Here's how the part is built. I have some questions about the finished solid (model axes, mm). A direction names the side the tool comes from. Round coordinates to 2 decimals unless told otherwise and drop trailing zeros. Order: outer loops, then holes, each group sorted by start corner. A loop starts at its lowest first (then second) coordinate and runs counter-clockwise, first axis right, second up. Notation, with made-up numbers: M 52.5,60.5 L 110.5,60.5 A16 cw 110.5,83.5 Z; hole C 52.5,70.5 d9. An arc over 180 degrees is marked long. Use one line per item in the form item = value. Start each with the question number.
```python
from build123d import *

# Parameters (mm, degrees)
BOSS_EXTRUDE1_DEPTH = 42
SKETCH2_R           = 2
CUT_EXTRUDE2_DEPTH  = 52.578217301
CUT_EXTRUDE3_DEPTH  = 4
SKETCH4_R           = 2
CUT_EXTRUDE4_DEPTH  = 52.578217301
SKETCH5_R           = 2
CUT_EXTRUDE5_DEPTH  = 65.722484597


with BuildPart() as part:
    # Sketch1 → Boss-Extrude1 (new body)
    with BuildSketch(Plane(origin=(0, 0, 0), x_dir=(0, 0, -1), z_dir=(1, 0, 0))):
        with BuildLine():
            Line((-0.25, 9.996874512), (-0.25, 22.5))
            Line((-0.25, 22.5), (-15, 22.5))
            ThreePointArc((-15, 22.5), (-18.535533906, 21.035533906), (-20, 17.5))
            Line((-20, 17.5), (-20, -17.5))
            ThreePointArc((-20, -17.5), (-18.535533906, -21.035533906), (-15, -22.5))
            Line((-15, -22.5), (-0.25, -22.5))
            Line((-0.25, -22.5), (-0.25, -9.996874512))
            ThreePointArc((-0.25, -9.996874512), (-10, 0), (-0.25, 9.996874512))
        make_face()
    extrude(amount=-BOSS_EXTRUDE1_DEPTH)

    # Sketch2 → Cut-Extrude2 (cut, through all)
    with BuildSketch(Plane.XY.offset(0.25)):
        with Locations(Location((-10.5, 13, 0), (0, 0, 90))):
            Circle(SKETCH2_R)
        with Locations(Location((-31.5, 13, 0), (0, 0, 90))):
            Circle(SKETCH2_R)
        with Locations(Location((-31.5, -13, 0), (0, 0, 90))):
            Circle(SKETCH2_R)
        with Locations(Location((-10.5, -13, 0), (0, 0, 90))):
            Circle(SKETCH2_R)
    extrude(amount=CUT_EXTRUDE2_DEPTH, mode=Mode.SUBTRACT)

    # Sketch3 → Cut-Extrude3 (cut)
    with BuildSketch(Plane.XY.offset(20)):
        with BuildLine():
            Line((-38, 13), (-38, 22.5))
            Line((-38, 22.5), (-25, 22.5))
            Line((-25, 22.5), (-25, 13))
            ThreePointArc((-25, 13), (-31.5, 6.5), (-38, 13))
        make_face()
        with BuildLine():
            Line((-17, 13), (-17, 22.5))
            Line((-17, 22.5), (-4, 22.5))
            Line((-4, 22.5), (-4, 13))
            ThreePointArc((-4, 13), (-10.5, 6.5), (-17, 13))
        make_face()
        with BuildLine():
            Line((-4, -22.5), (-4, -13))
            ThreePointArc((-4, -13), (-10.5, -6.5), (-17, -13))
            Line((-17, -13), (-17, -22.5))
            Line((-17, -22.5), (-4, -22.5))
        make_face()
        with BuildLine():
            Line((-25, -22.5), (-25, -13))
            ThreePointArc((-25, -13), (-31.5, -6.5), (-38, -13))
            Line((-38, -13), (-38, -22.5))
            Line((-38, -22.5), (-25, -22.5))
        make_face()
    extrude(amount=-CUT_EXTRUDE3_DEPTH, mode=Mode.SUBTRACT)

    # Sketch4 → Cut-Extrude4 (cut, through all)
    with BuildSketch(Plane.XY.offset(20)):
        with Locations((-10.5, 0)):
            Circle(SKETCH4_R)
        with Locations((-31.5, 0)):
            Circle(SKETCH4_R)
    extrude(amount=-CUT_EXTRUDE4_DEPTH, mode=Mode.SUBTRACT)

    # Sketch5 → Cut-Extrude5 (cut, through all)
    with BuildSketch(Plane.XZ.offset(22.5)):
        with Locations(Location((-21, 13, 0), (0, 0, 90))):
            Circle(SKETCH5_R)
    extrude(amount=-CUT_EXTRUDE5_DEPTH, mode=Mode.SUBTRACT)


solid = part.part
```
1) On a 3-axis mill with a long thin cutter (end or side, diameter ignored), from which of +Z, -Z, +X, -X, +Y, -Y can I reach the whole of each face in a straight line? I mean faces 4 (the flat face through (-10, 16, 16)), 5 (the cylindrical face through (-20.706, -21.564, 17.913)), 6 (the flat face through (-17, -18, 18)). Say none if no direction works.
2) Will these pins go through, and if not, where does the flat tip stop? pin 1 Ø4 at (x, y) = (-13.5, 14) entering from +Z; pin 2 Ø2.5 at (x, z) = (-21, 13) entering from +Y; pin 3 Ø5 at (x, y) = (-10.5, 0) entering from -Z; pin 4 Ø6.5 at (x, y) = (-31.5, 0) entering from -Z.
3) If we mould it in two halves opening along Z, with no side actions, what happens to faces 1 (the cylindrical face through (-23, 0, 13)), 2 (the cylindrical face through (-31.4, -6.5, 18)), 3 (the flat face through (-32, -16, 16))? For each: +Z half, -Z half, draft (parallel to the pull), parting line (faces both ways), or undercut.
4) If I drill on line 1 (X direction, y = 18.5, z = 18); line 2 (X direction, y = 13, z = 8.5); line 3 (Y direction, x = -31.5, z = 14), over which ranges is the centre line in solid material (lowest first)?
5) If we section it at B-B on y = -1: Write out the boundary of the cut face in (x, z), then the cut area to 3 significant figures.
6) If we section it at D-D on y = -9: Write out the boundary of the cut face in (x, z), then the cut area to 3 significant figures.
7) If we section it at C-C on z = 3.25: Write out the boundary of the cut face in (x, y).
8) If we section it at A-A on x = -10.5: Write out the boundary of the cut face in (y, z).
Completed:
q1.face_4 = +Z, +Y
q1.face_5 = +Z, +X, -X, -Y
q1.face_6 = +Z, -Y
q2.pin_1 = 16
q2.pin_2 = through
q2.pin_3 = 9.68
q2.pin_4 = 9.46
q3.face_1 = undercut
q3.face_2 = draft
q3.face_3 = +Z half
q4.line_1 = -42 to -38, -25 to -17, -4 to 0
q4.line_2 = -42 to -33.5, -29.5 to -12.5, -8.5 to 0
q4.line_3 = -22.5 to -15, -11 to -2, 2 to 11, 15 to 22.5
q5.outline = M -42,9.95 L -33.23,9.95 L -33.23,20 L -42,20 Z; M -29.77,9.95 L -12.23,9.95 L -12.23,20 L -29.77,20 Z; M -8.77,9.95 L 0,9.95 L 0,20 L -8.77,20 Z; hole C -21,13 d4
q5.area = 340 mm²
q6.outline = M -42,4.36 L 0,4.36 L 0,20 L -5.38,20 L -5.38,16 L -15.62,16 L -15.62,20 L -26.38,20 L -26.38,16 L -36.62,16 L -36.62,20 L -42,20 Z; hole C -21,13 d4
q6.area = 562 mm²
q7.outline = M -42,-22.5 L 0,-22.5 L 0,-9.46 L -42,-9.46 Z; M -42,9.46 L 0,9.46 L 0,22.5 L -42,22.5 Z; hole C -31.5,-13 d4; hole C -31.5,13 d4; hole C -10.5,-13 d4; hole C -10.5,13 d4
q8.outline = M -22.5,0.25 L -15,0.25 L -15,16 L -22.4,16 A5 ccw -22.5,15 Z; M -11,0.25 L -10,0.25 A10 cw -2,9.8 L -2,20 L -6.5,20 L -6.5,16 L -11,16 Z; M 2,9.8 A10 cw 10,0.25 L 11,0.25 L 11,16 L 6.5,16 L 6.5,20 L 2,20 Z; M 15,0.25 L 22.5,0.25 L 22.5,15 A5 ccw 22.4,16 L 15,16 Z
